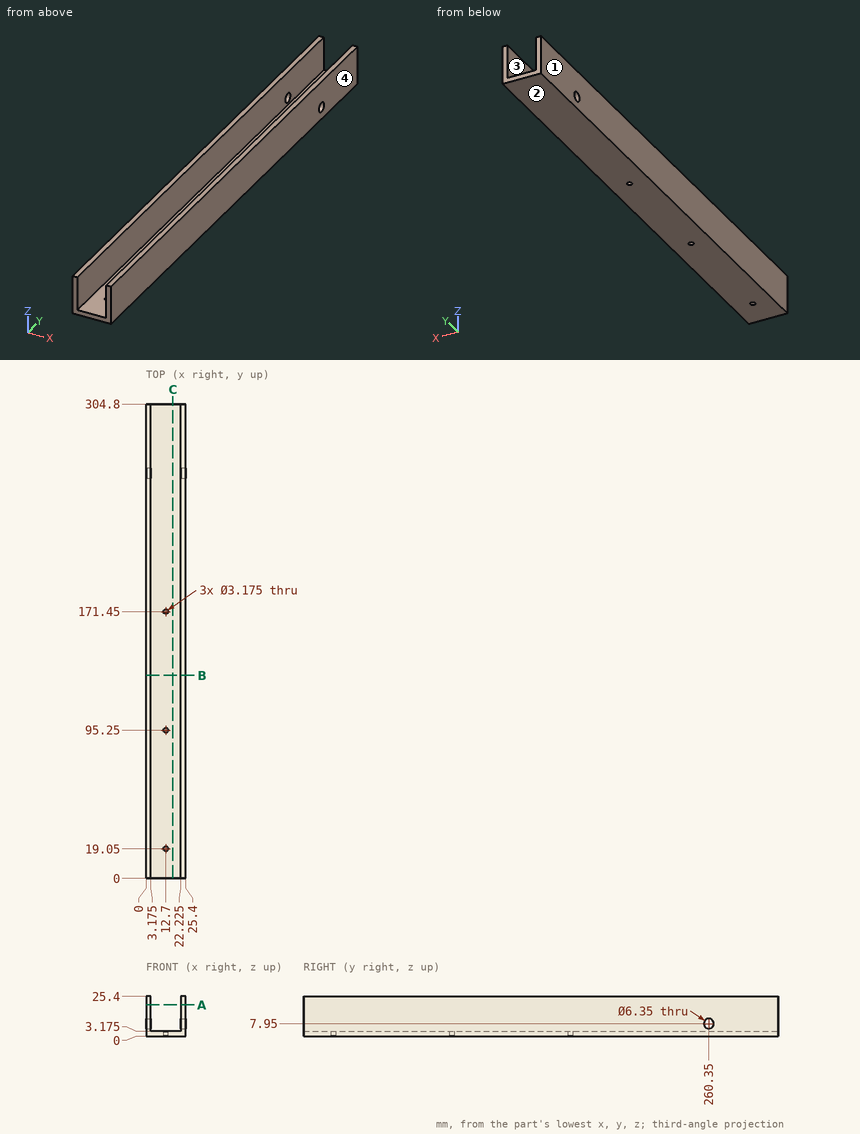
Input: dimensioned drawing with shaded views. Units: mm. Origin: part minimum x, y, z. Coordinates: 2 decimals unless noted, no trailing zeros. Loops run counter-clockwise (first coordinate to the right, second up) from the corner with the lowest first, then second, coordinate; pieces in that order, holes last. Notation, with made-up numbers: M 70,82 L 108,82 A17 ccw 108,107 Z; hole C -4,23 d11. An arc over 180 degrees is marked long. One line per item, written item: value.
(1) Section A-A (z = 20). Output: boundary loops of the cut face in (x, y) (3 decimals).
Filled in:
outline: M 0,0 L 3.175,0 L 3.175,304.8 L 0,304.8 Z; M 22.225,0 L 25.4,0 L 25.4,304.8 L 22.225,304.8 Z
(2) Section C-C (x = 17.25). Output: boundary loops of the cut face in (y, z) (3 decimals).
Filled in:
outline: M 0,0 L 304.8,0 L 304.8,3.175 L 0,3.175 Z
(3) Pull-direction query (X, two-part tool) for the marked faces 1, 2, 3 and 4; classes: +X half, -X half, draft (parallel to the pull), parting line (faces both ways), or undercut.
Filled in:
face 1: -X half
face 2: draft
face 3: undercut
face 4: +X half
(4) Section B-B (y = 130.5). Output: boundary loops of the cut face in (x, z) (3 decimals), and give its area (3 significant figures).
Filled in:
outline: M 0,0 L 25.4,0 L 25.4,25.4 L 22.225,25.4 L 22.225,3.175 L 3.175,3.175 L 3.175,25.4 L 0,25.4 Z
area: 222 mm^2
(5) Line query: line 1 along Y through (x, z) = (12.7, 2.4); line 2 along X through (y, z) = (196.5, 16.5) (3 decimals); line 3 along X through (y, z) = (95.25, 1.35). Output: solid intervals per line, ascending. Write a range as from..to.
Filled in:
line 1: 0..17.46, 20.64..93.66, 96.84..169.86, 173.04..304.8
line 2: 0..3.175, 22.225..25.4
line 3: 0..11.11, 14.29..25.4
(6) Pin query (flat end, axial travel): pin 1 (5 mm diameter, centred on x = 12.7, y = 171.45, fed in from +Z) (3 decimals). Return the tip coordinate at first contact, or that it passes through.
Filled in:
pin 1: z = 3.175
